```python
from build123d import *
from build123d.topology import SkipClean

# Parameters (mm, degrees)
BOSS_EXTRUDE1_DEPTH     = 8.55
SKETCH2_W               = 10.7
SKETCH2_H               = 10.8
CUT_EXTRUDE1_DEPTH      = 17
SKETCH3_R               = 6
BOSS_EXTRUDE2_DEPTH     = 18
SKETCH4_R               = 4.2
CUT_EXTRUDE2_DEPTH      = 25.239275979
BOSS_EXTRUDE5_DEPTH     = 17.1
SKETCH7_R               = 2.2
CUT_EXTRUDE3_DEPTH      = 40.626944786
CUT_EXTRUDE4_REACH      = 33.94
SKETCH10_W              = 8.106
SKETCH10_H              = 1.5
SKETCH11_W              = 6.997
SKETCH11_H              = 1
CUT_EXTRUDE5_DEPTH      = 27.591587091
CUT_EXTRUDE6_REACH      = 42.967
CUT_EXTRUDE6_END_RADIUS = 6
CUT_EXTRUDE7_START      = -16.8
CUT_EXTRUDE7_DEPTH      = 16.8
BOSS_EXTRUDE6_DEPTH     = 1.553
BOSS_EXTRUDE7_REACH     = 36.128
CUT_EXTRUDE8_REACH      = 43.851
CUT_EXTRUDE9_REACH      = 43.851


with BuildPart() as part:
    # Sketch1 → Boss-Extrude1 (new, symmetric)
    with BuildSketch(Plane(origin=(0, 0, 0), x_dir=(0, 0, -1), z_dir=(1, 0, 0))):
        Polygon((0, 0), (0, -3), (-16.0587, -13.8), (-35, -13.8), (-35, 0), align=None)
    extrude(amount=BOSS_EXTRUDE1_DEPTH, both=True)

    # Sketch2 → Cut-Extrude1 (cut)
    with BuildSketch(Plane.XY.offset(35)):
        with Locations((0, -5.4)):
            Rectangle(SKETCH2_W, SKETCH2_H)
    extrude(amount=-CUT_EXTRUDE1_DEPTH, mode=Mode.SUBTRACT)

    # Sketch3 → Boss-Extrude2 (add, through all)
    with BuildSketch(Plane.XY.offset(18)):
        with Locations((0, -0.30175)):
            Circle(SKETCH3_R)
    extrude(amount=-BOSS_EXTRUDE2_DEPTH)

    # Sketch4 → Cut-Extrude2 (cut, through all)
    with BuildSketch(Plane.XY.offset(18)):
        with Locations((0, -0.30175)):
            Circle(SKETCH4_R)
    extrude(amount=-CUT_EXTRUDE2_DEPTH, mode=Mode.SUBTRACT)

    # Sketch8 → Boss-Extrude5 (add, through all)
    with BuildSketch(Plane(origin=(8.55, 0, 0), x_dir=(0, 0, -1), z_dir=(1, 0, 0))):
        Polygon((-26.702, -13.8), (-26.702, -15.3), (-25.702, -15.3), (-24.202, -13.8), align=None)
        Polygon((-16.0587, -13.8), (-15.002, -13.8), (-15.002, -14.8), (-14.002, -14.8), (-13, -13.8), (-11.045997115, -10.428793666), align=None)
    extrude(amount=-BOSS_EXTRUDE5_DEPTH)

    # Sketch7 → Cut-Extrude3 (cut, through all)
    with BuildSketch(Plane(origin=(0, -10.8, 0), x_dir=(1, 0, 0), z_dir=(0, 1, 0))):
        with Locations(Location((0, -25, 0), (0, 0, 180))):
            Circle(SKETCH7_R)
    extrude(amount=-CUT_EXTRUDE3_DEPTH, mode=Mode.SUBTRACT)

    # Cut-Extrude4: up to this plane
    cut_extrude4_end = Plane(origin=(-8.55, -15.3, 25.702), z_dir=(0, -0.7071067811865471, -0.707106781186548))
    # Sketch10 → Cut-Extrude4 (cut, up to the surface)
    with BuildSketch(Plane.XY.offset(26.702), mode=Mode.PRIVATE) as cut_extrude4_sk1:
        with Locations((0, -14.55)):
            Rectangle(SKETCH10_W, SKETCH10_H)
    cut_extrude4_tool1 = split(extrude(cut_extrude4_sk1.sketch, amount=-CUT_EXTRUDE4_REACH, mode=Mode.PRIVATE), bisect_by=cut_extrude4_end, keep=Keep.BOTH, mode=Mode.PRIVATE)
    add(cut_extrude4_tool1.solids().sort_by_distance((0, -14.55, 26.702))[0], mode=Mode.SUBTRACT)

    # Sketch11 → Cut-Extrude5 (cut, through all)
    with BuildSketch(Plane.XY.offset(15.002)):
        with Locations((-5.0515, -14.3)):
            Rectangle(SKETCH11_W, SKETCH11_H)
        with Locations((5.0515, -14.3)):
            Rectangle(SKETCH11_W, SKETCH11_H)
    extrude(amount=-CUT_EXTRUDE5_DEPTH, mode=Mode.SUBTRACT)

    # Cut-Extrude6: up to this cylinder (the profile starts outside it)
    cut_extrude6_end = Plane(origin=(0, -0.30175, 7.230062), z_dir=(0, 0, 1)) * Cylinder(CUT_EXTRUDE6_END_RADIUS, 98.934, mode=Mode.PRIVATE)
    # Sketch12 → Cut-Extrude6 (cut, up to the surface)
    with BuildSketch(Plane.XZ.offset(13.8), mode=Mode.PRIVATE) as cut_extrude6_sk1:
        Polygon((-1.553, 13), (-5.353, 16.8), (-5.353, 0), (5.353, 0), (5.353, 16.8), (1.553, 13), align=None)
    cut_extrude6_tool1 = extrude(cut_extrude6_sk1.sketch, amount=-CUT_EXTRUDE6_REACH, mode=Mode.PRIVATE) - cut_extrude6_end
    add(cut_extrude6_tool1.solids().sort_by_distance((0, -13.8, 7.230062))[0], mode=Mode.SUBTRACT)

    # Sketch13 → Cut-Extrude7 (cut)
    with SkipClean():  # the faces are left unmerged after this step: merging them gives an invalid solid
        with BuildSketch(Plane(origin=(0, 0, 0), x_dir=(-1, 0, 0), z_dir=(0, 0, -1)).offset(CUT_EXTRUDE7_START)):
            with BuildLine():
                Line((-5.359052802, -3), (-5.353, -10.428793666))
                Line((-5.353, -10.428793666), (5.353, -10.428793666))
                Line((5.353, -10.428793666), (5.359052802, -3))
                ThreePointArc((5.359052802, -3), (0, -6.30175), (-5.359052802, -3))
            make_face()
        extrude(amount=CUT_EXTRUDE7_DEPTH, mode=Mode.SUBTRACT)

    # Sketch14 → Boss-Extrude6 (add, symmetric)
    with SkipClean():  # the faces are left unmerged after this step: merging them gives an invalid solid
        with BuildSketch(Plane(origin=(0, 0, 0), x_dir=(0, 0, -1), z_dir=(1, 0, 0))):
            Polygon((-13, -13.8), (-8.073269662, -5.3), (-16.8, -5.3), (-16.8, -13.8), align=None)
        extrude(amount=BOSS_EXTRUDE6_DEPTH, both=True)

    # Sketch15 → Boss-Extrude7 (add, up to next)
    with BuildSketch(Plane(origin=(-7.436377386, -6.523873454, 7.436377386), x_dir=(-0.7993387140757535, 0.3962687040508023, -0.4516953999872244), z_dir=(0.6008807037838052, 0.5271477588310114, -0.6008807037838052)), mode=Mode.PRIVATE) as boss_extrude7_sk1:
        Polygon((-11.246017774, 0.733681451), (-11.246017774, 6.495798547), (-15.999947407, 3.239704803), align=None)
    boss_extrude7_tool1 = extrude(boss_extrude7_sk1.sketch, amount=-BOSS_EXTRUDE7_REACH, mode=Mode.PRIVATE) - part.part
    boss_extrude7 = boss_extrude7_tool1.solids().sort_by_distance((2.819667, -8.984956, 15.533333))[0]
    add(boss_extrude7)

    # Mirror1: Boss-Extrude7 across plane
    with SkipClean():  # the faces are left unmerged after this step: merging them gives an invalid solid
        add(boss_extrude7.mirror(Plane(origin=(0, 0, 0), x_dir=(0, 0, 1), z_dir=(1, 0, 0))))

    # Sketch16 → Cut-Extrude8 (cut, up to next)
    with BuildSketch(Plane(origin=(8.55, 0, 0), x_dir=(0, 0, -1), z_dir=(1, 0, 0)), mode=Mode.PRIVATE) as cut_extrude8_sk1:
        Polygon((-11.045997115, -10.428793666), (-16.0587, -13.8), (-13, -13.8), align=None)
    cut_extrude8_tool1 = extrude(cut_extrude8_sk1.sketch, amount=-CUT_EXTRUDE8_REACH, mode=Mode.PRIVATE) & part.part
    add(cut_extrude8_tool1.solids().sort_by_distance((8.55, -12.676265, 13.368232))[0], mode=Mode.SUBTRACT)

    # Sketch17 → Cut-Extrude9 (cut, up to next)
    with BuildSketch(Plane.ZY.offset(8.55), mode=Mode.PRIVATE) as cut_extrude9_sk1:
        Polygon((11.045997115, -10.428793666), (16.0587, -13.8), (13, -13.8), align=None)
    cut_extrude9_tool1 = extrude(cut_extrude9_sk1.sketch, amount=-CUT_EXTRUDE9_REACH, mode=Mode.PRIVATE) & part.part
    add(cut_extrude9_tool1.solids().sort_by_distance((-8.55, -12.676265, 13.368232))[0], mode=Mode.SUBTRACT)


solid = part.part
```
Verification items for the finished model (mm, model axes). A direction names the side the tool comes from. Give positions to 0.01 mm unless a question says otherwise; leave off trailing zeros. Write each loop counter-clockwise with the first axis right and the second up, starting at its lowest first coordinate (ties: lowest second). Pieces come first, ordered by that corner, then holes. Notation, with made-up numbers: M 82,81 L 131,81 A17 ccw 131,90 Z; hole C 80,40.5 d4. An arc over 180 degrees is marked long. One line per question, with ' | ' between items.
1) Section check A-A on z = 21.5. Enter the section's corners in (x, y).
Result:
outline: M -8.55,-13.8 L 8.55,-13.8 L 8.55,0 L 5.35,0 L 5.35,-10.8 L -5.35,-10.8 L -5.35,0 L -8.55,0 Z
2) Set-up check for faces 1 (the flat face through (0, -14, 15.002)), 2 (the flat face through (0, -10.8, 29)), 3 (the flat face through (1.553, -8, 13)), 4 (the flat face through (4.053, -14, 26)): record each of +Z, -Z, +X, -X, +Y, -Y from which the full face is reachable in a straight line by a thin tool's end or side.
Result:
face 1: +Z, +X, -X, -Y | face 2: +Z, +Y | face 3: -Z | face 4: +Z, -Z, -Y
3) Section check D-D on y = -9. Enter the section's corners in (x, z), plus the area to 3 significant figures.
Result:
outline: M -8.55,8.92 L -5.35,8.92 L -5.35,16.8 L -4.1,16.8 L -1.55,14.25 L -1.55,10.22 L 1.55,10.22 L 1.55,14.25 L 4.1,16.8 L 5.35,16.8 L 5.35,8.92 L 8.55,8.92 L 8.55,35 L 5.35,35 L 5.35,18 L -5.35,18 L -5.35,35 L -8.55,35 Z | area: 207 mm2
4) Gauge pin test, flat ends, axial feed: pin 1 Ø4 at (x, z) = (0, 25) entering from -Y; pin 2 Ø5.5 at (x, z) = (2, 27.5) entering from +Y; pin 3 Ø1.2 at (x, y) = (7, -14.5) entering from +Z; pin 4 Ø2 at (x, z) = (-5.5, 13) entering from -Y. Record the tip position at first contact, or that the pin passes through.
Result:
pin 1: passes through | pin 2: stops at y = -10.8 | pin 3: stops at z = 26.7 | pin 4: stops at y = -12.42
5) Mould release check, pull along X, two halves, no side actions. Record for faces 5 (the cylindrical face through (0.128, 5.697, 9.126)), 6 (the flat face through (5.35, -5, 27)), 7 (the flat face through (6, -15, 26.702)): released by +X, released by -X, zero draft, split by the parting line, or undercut.
Result:
face 5: split by the parting line | face 6: undercut | face 7: zero draft
6) Section check C-C on z = 25. Enter the section's corners in (x, y).
Result:
outline: M -8.55,-14.6 L -4.05,-14.6 L -4.05,-13.8 L -2.2,-13.8 L -2.2,-10.8 L -5.35,-10.8 L -5.35,0 L -8.55,0 Z; M 2.2,-13.8 L 4.05,-13.8 L 4.05,-14.6 L 8.55,-14.6 L 8.55,0 L 5.35,0 L 5.35,-10.8 L 2.2,-10.8 Z
7) Thickness scan on line 1 along X through (y, z) = (-5.75, 8); line 2 along X through (y, z) = (-4, 30); line 3 along Y through (x, z) = (0, 6.75). Record the ranges inside material, lowest first. Write a range as [from, to].
Result:
line 1: x = [-8.55, -5.36], [-2.51, 2.51], [5.36, 8.55] | line 2: x = [-8.55, -5.35], [5.35, 8.55] | line 3: y = [-6.3, -4.5], [3.9, 5.7]
8) Section check B-B on x = 0. Enter the section's corners in (y, z).
Result:
outline: M -14.8,14 L -13.8,13 L -6.3,8.65 L -6.3,0 L -4.5,0 L -4.5,18 L -10.8,18 L -10.8,22.8 L -13.8,22.8 L -13.8,15 L -14.8,15 Z; M -13.8,27.2 L -10.8,27.2 L -10.8,35 L -13.8,35 Z; M 3.9,0 L 5.7,0 L 5.7,18 L 3.9,18 Z
